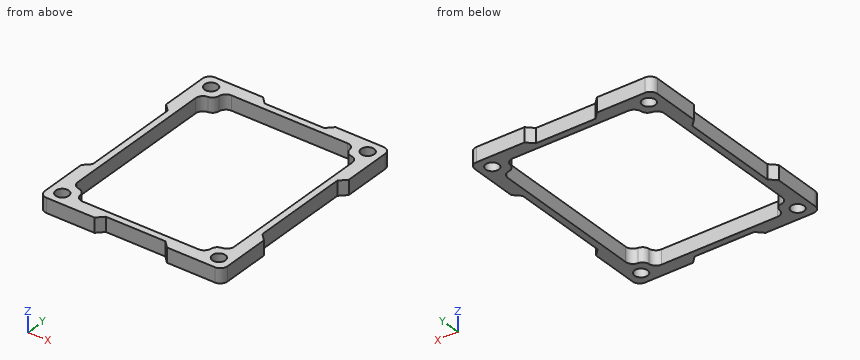
Autodesk Inventor part; units mm, degrees
ref_plane "YZ Plane" through (0, 0, 0) normal (1, 0, 0) x (0, 1, 0)
ref_plane "XZ Plane" through (0, 0, 0) normal (0, 1, 0) x (-1, 0, 0)
ref_plane "XY Plane" through (0, 0, 0) normal (0, 0, 1) x (1, 0, 0)
sketch "Sketch1" plane through (0, 0, 0) normal (0, 0, 1) x (1, 0, 0)
  line L0 (0, 18) -> (0, 0)
  line L1 (0, 0) -> (18, 0)
  line L2 (18, 0) -> (18, 18)
  line L3 (18, 18) -> (0, 18)
  circle A0 centre (9, 9) radius 4.5
  line L4 (0, 153) -> (18, 153)
  line L5 (0, 135) -> (0, 153)
  line L6 (18, 135) -> (0, 135)
  line L7 (18, 153) -> (18, 135)
  line L8 (0, 153) -> (18, 153)
  circle A1 centre (9, 144) radius 4.5
  line L9 (126, 135) -> (126, 153)
  line L10 (126, 153) -> (108, 153)
  line L11 (108, 153) -> (108, 135)
  line L12 (108, 135) -> (126, 135)
  circle A2 centre (117, 144) radius 4.5
  line L13 (126, 18) -> (126, 0)
  line L14 (108, 18) -> (126, 18)
  line L15 (108, 0) -> (108, 18)
  line L16 (126, 0) -> (108, 0)
  circle A3 centre (117, 9) radius 4.5
  line L17 (18, 0) -> (108, 0)
  line L18 (108, 0) -> (108, 9)
  line L19 (108, 9) -> (18, 9)
  line L20 (18, 9) -> (18, 0)
  line L21 (126, 18) -> (117, 18)
  line L22 (117, 18) -> (117, 135)
  line L23 (117, 135) -> (126, 135)
  line L24 (126, 135) -> (126, 18)
  line L25 (108, 153) -> (18, 153)
  line L26 (18, 153) -> (18, 144)
  line L27 (18, 144) -> (108, 144)
  line L28 (108, 144) -> (108, 153)
  line L29 (0, 135) -> (9, 135)
  line L30 (9, 135) -> (9, 18)
  line L31 (9, 18) -> (0, 18)
  line L32 (0, 18) -> (0, 135)
  line L33 (126, 115) -> (121.5, 115)
  line L34 (121.5, 115) -> (121.5, 38)
  line L35 (121.5, 38) -> (126, 38)
  line L36 (126, 38) -> (126, 115)
  line L37 (88, 0) -> (38, 0)
  line L38 (38, 0) -> (38, 4.5)
  line L39 (38, 4.5) -> (88, 4.5)
  line L40 (88, 4.5) -> (88, 0)
  line L41 (0, 38) -> (4.5, 38)
  line L42 (4.5, 38) -> (4.5, 115)
  line L43 (4.5, 115) -> (0, 115)
  line L44 (0, 115) -> (0, 38)
  line L45 (38, 153) -> (88, 153)
  line L46 (88, 153) -> (88, 148.5)
  line L47 (88, 148.5) -> (38, 148.5)
  line L48 (38, 148.5) -> (38, 153)
  point P0 (18, 9)
  point P1 (38, 0)
  dimension "d0" = 9
  dimension "d1" = 9
  dimension "d2" = 9
  dimension "d3" = 9
  dimension "d4" = 4.5
  dimension "d5" = 4.5
  dimension "d6" = 4.5
  dimension "d7" = 4.5
  dimension "d8" = 20
  dimension "d9" = 20
  dimension "d10" = 20
  dimension "d11" = 20
  dimension "d12" = 20
  dimension "d13" = 20
  dimension "d14" = 20
  dimension "d15" = 20
extrude "Extrusion1" add sketch "Sketch1" along normal blind 10 contours L3 L2 L1 L0 | L32 L41 L42 L43 L6 L30 L3 | L2 L19 L15 L17 L40 L39 L38 | L6 L5 L4 L7 | L15 L14 L13 L16 | L7 L25 L48 L47 L46 L11 L27 | L11 L10 L9 L12 | L22 L12 L24 L33 L34 L35 L14
fillet "Fillet1" radius 5 16 edges at (108, 144, 5) (117, 135, 5) (108, 135, 5) (18, 144, 5) (18, 135, 5) (9, 135, 5) (9, 18, 5) (18, 18, 5) (18, 9, 5) (108, 9, 5) (108, 18, 5) (117, 18, 5) (0, 153, 5) (126, 153, 5) (126, 0, 5) (0, 0, 5)
chamfer "Chamfer1" distance 4.5 angle 45 8 edges at (38, 148.5, 5) (88, 148.5, 5) (121.5, 115, 5) (121.5, 38, 5) (38, 4.5, 5) (88, 4.5, 5) (4.5, 38, 5) (4.5, 115, 5)
equation "\"d1\" = d0"
equation "\"d2\" = d0"
equation "\"d3\" = d0"
equation "\"d4\" = 0.5 * d0"
equation "\"d5\" = 0.5 * d0"
equation "\"d6\" = 0.5 * d0"
equation "\"d7\" = 0.5 * d0"
equation "\"d9\" = d8"
equation "\"d10\" = d8"
equation "\"d11\" = d8"
equation "\"d12\" = d8"
equation "\"d13\" = d8"
equation "\"d14\" = d8"
equation "\"d15\" = d8"
properties part number "Servo-Gear-MountingPlate"
Read the model definition and answer for the solid it produces. Units are mm, in the model's axes. Coordinates: 2 decimals unless noted, no trailing zeros. Loops run counter-clockwise (first coordinate to the right, second up) from the corner with the lowest first, then second, coordinate; pieces in that order, holes last.
Q1. The part is cut by section B-B on y = 104. Write down the section's boundary in (x, z), and give its area (3 significant figures).
Q2. The part is cut by section C-C on z = 5.75. Give the number of separate pieces and of enclosed holes in the cut face, and give its area (3 significant figures).
Q3. The part is cut by section A-A on x = 67. Write down the section's boundary in (y, z), and give its area (3 significant figures).
Q4. Each of these flat-tipped pins is pushed along its axis until it touches: pin 1 Ø2 at (y, z) = (111.5, 4.5) entering from +X; pin 2 Ø5 at (x, z) = (61, 7) entering from -Y; pin 3 Ø5.5 at (x, y) = (9, 144) entering from +Z; pin 4 Ø3 at (y, z) = (93.5, 4.5) entering from +X. Where does it stop, or does it pass through?
Q5. Consider probe 1 along X at (y, z) = (88.5, 9.25); probe 2 along X at (y, z) = (31, 1.5); probe 3 along Y at (x, z) = (118, 5.75). Determine where each line is inside the solid, lowest interval first.
Results below:
1. outline: (4.5, 0) - (9, 0) - (9, 10) - (4.5, 10) - close; (117, 0) - (121.5, 0) - (121.5, 10) - (117, 10) - close
1. area: 90.0 mm2
2. separate pieces: 1
2. enclosed holes: 5
2. area: 3,710 mm2
3. outline: (4.5, 0) - (9, 0) - (9, 10) - (4.5, 10) - close; (144, 0) - (148.5, 0) - (148.5, 10) - (144, 10) - close
3. area: 90.0 mm2
4. pin 1: stops at x = 123.5
4. pin 2: stops at y = 4.5
4. pin 3: passes through
4. pin 4: stops at x = 121.5
5. probe 1: x = 4.5 to 9, 117 to 121.5
5. probe 2: x = 0 to 9, 117 to 126
5. probe 3: y = 0 to 4.61, 13.39 to 139.61, 148.39 to 153
